```python
from build123d import *

# Parameters (mm, degrees)
DODANIE_WYCI_GNI_CIE1_DEPTH = 3
OTWORY_USTALAJ_CE_12_0MM1_D = 12


with BuildPart() as part:
    # Szkic1 → Dodanie-wyciągnięcie1 (new body)
    with BuildSketch(Plane.XY):
        with BuildLine():
            Line((-120, -105), (120, -105))
            ThreePointArc((120, -105), (155.355339059, -90.355339059), (170, -55))
            Line((170, -55), (170, 55))
            ThreePointArc((170, 55), (155.355339059, 90.355339059), (120, 105))
            Line((120, 105), (-120, 105))
            ThreePointArc((-120, 105), (-155.355339059, 90.355339059), (-170, 55))
            Line((-170, 55), (-170, -55))
            ThreePointArc((-170, -55), (-155.355339059, -90.355339059), (-120, -105))
        make_face()
    extrude(amount=DODANIE_WYCI_GNI_CIE1_DEPTH)

    # Otwory ustalające Ø12.0mm1 (through all)
    with Locations(Plane(origin=(0, 0, 0), x_dir=(-1, 0, 0), z_dir=(0, 0, -1))):
        with Locations((45, 45), (-45, 45), (45, -45), (-45, -45), (-150, 0), (150, 0)):
            Hole(OTWORY_USTALAJ_CE_12_0MM1_D / 2)


solid = part.part
```
The listing builds one solid part. Answer for the finished solid, in the listing's coordinates (mm). Round coordinates to 2 decimals unless told otherwise and drop trailing zeros. Loops run counter-clockwise (first coordinate to the right, second up) from the corner with the lowest first, then second, coordinate; pieces in that order, holes last. Notation, with made-up numbers: (-35.5, 86) - (-15.5, 86) arc R20 ccw to (-15.5, 100) - close; hole circle Ø3 at (-36.5, -39.5). An arc over 180 degrees is marked (long way). Return JSON: item names as keys, results as strings. Group by question number.
1. The part is cut by section D-D on x = 150. Determine the outline of the cut face in (y, z).
2. The part is cut by section B-B on x = -45. Determine the outline of the cut face in (y, z), then the cut area to 3 significant figures.
3. The mould has two halves that part along Y. Classify faces 1 (the flat face through (-2, 1, 3)), 2 (the cylindrical face through (-154.76, -3.65, 1.52)), 3 (the cylindrical face through (155.742, 89.964, 1.479)), 4 (the cylindrical face through (40.24, -48.65, 1.52)): pulls with the +Y half, pulls with the -Y half, needs draft (parallel to the pull), parting line crosses it, or undercut.
4. The part is cut by section A-A on y = 45. Determine the outline of the cut face in (x, z).
5. Consider probe 1 along Y at (x, z) = (-45, 2.15); probe 2 along X at (y, z) = (47.5, 0.7); probe 3 along X at (y, z) = (3, 2.2). Determine where each line is inside the solid, lowest interval first.
6. The part is cut by section C-C on z = 2.3. Determine the outline of the cut face in (x, y), then the cut area to 3 significant figures.
Resolved:
{
 "1": {"outline": "(-95, 0) - (-6, 0) - (-6, 3) - (-95, 3) - close; (6, 0) - (95, 0) - (95, 3) - (6, 3) - close"},
 "2": {"outline": "(-105, 0) - (-51, 0) - (-51, 3) - (-105, 3) - close; (-39, 0) - (39, 0) - (39, 3) - (-39, 3) - close; (51, 0) - (105, 0) - (105, 3) - (51, 3) - close", "area": "558 mm²"},
 "3": {"face 1": "needs draft", "face 2": "undercut", "face 3": "pulls with the +Y half", "face 4": "undercut"},
 "4": {"outline": "(-170, 0) - (-51, 0) - (-51, 3) - (-170, 3) - close; (-39, 0) - (39, 0) - (39, 3) - (-39, 3) - close; (51, 0) - (170, 0) - (170, 3) - (51, 3) - close"},
 "5": {"probe 1": "y = -105 to -51, -39 to 39, 51 to 105", "probe 2": "x = -170 to -50.45, -39.55 to 39.55, 50.45 to 170", "probe 3": "x = -170 to -155.2, -144.8 to 144.8, 155.2 to 170"},
 "6": {"outline": "(-170, -55) arc R50 ccw to (-120, -105) - (120, -105) arc R50 ccw to (170, -55) - (170, 55) arc R50 ccw to (120, 105) - (-120, 105) arc R50 ccw to (-170, 55) - close; hole circle Ø12 at (-150, 0); hole circle Ø12 at (-45, -45); hole circle Ø12 at (-45, 45); hole circle Ø12 at (45, -45); hole circle Ø12 at (45, 45); hole circle Ø12 at (150, 0)", "area": "68,600 mm²"}
}
